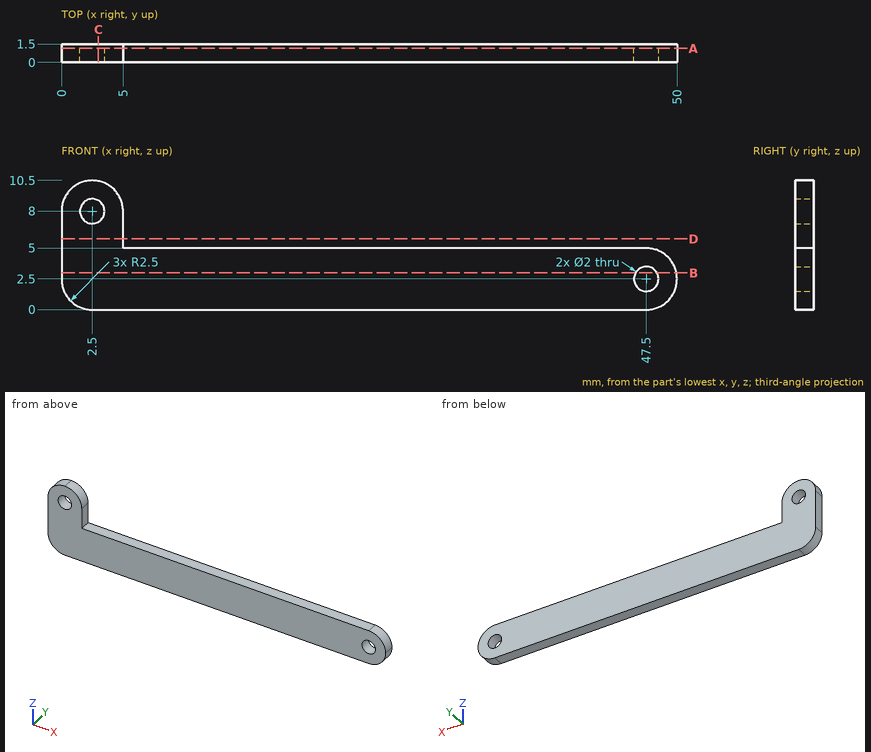
Here's the drawing with two shaded views (mm, measured from the low corner). I have some questions. Give positions to 0.01 mm unless a question says otherwise; leave off trailing zeros. Loops run counter-clockwise (first coordinate to the right, second up) from the corner with the lowest first, then second, coordinate; pieces in that order, holes last. Notation, with made-up numbers: M 14.25,11 L 37.25,11 A20 cw 37.25,45 Z; hole C 74,89.5 d9. An arc over 180 degrees is marked long. One line per item, written item: value.
1) Imagine slicing it at A-A on y = 1.15. Write out the boundary of the cut face in (x, z), and give its area (3 significant figures).
Geometry check:
outline: M 0,2.5 A2.5 ccw 2.5,0 L 47.5,0 A2.5 ccw 47.5,5 L 5,5 L 5,8 A2.5 ccw 0,8 Z; hole C 2.5,8 d2; hole C 47.5,2.5 d2
area: 265 mm²
2) I'm going to push a flat-ended pin straight in: pin 1 (0.8 mm diameter, centred on x = 28.5, y = 0.5, fed in from +Z). Where does the tip first touch, or does it pass through?
Geometry check:
pin 1: stops at z = 5
3) Imagine slicing it at B-B on z = 3. Write out the boundary of the cut face in (x, y), and give its area (3 significant figures).
Geometry check:
outline: M 0,0 L 46.63,0 L 46.63,1.5 L 0,1.5 Z; M 48.37,0 L 49.95,0 L 49.95,1.5 L 48.37,1.5 Z
area: 72.3 mm²
4) Imagine slicing it at C-C on x = 3. Write out the boundary of the cut face in (y, z), and give its area (3 significant figures).
Geometry check:
outline: M 0,0 L 1.5,0 L 1.5,7.13 L 0,7.13 Z; M 0,8.87 L 1.5,8.87 L 1.5,10.45 L 0,10.45 Z
area: 13.1 mm²
5) Please list where this line runs through material, in increasing order: line 1 (Z direction, x = 24, y = 0.65).
Geometry check:
line 1: z = 0 to 5
6) Imagine slicing it at D-D on z = 5.75. Write out the boundary of the cut face in (x, y), and give its area (3 significant figures).
Geometry check:
outline: M 0,0 L 5,0 L 5,1.5 L 0,1.5 Z
area: 7.50 mm²
